Can you work these out from the model? Positions are in its coordinate system, mm. A direction names the side the tool comes from. Round coordinates to 2 decimals unless told otherwise and drop trailing zeros. Write each loop counter-clockwise with the first axis right and the second up, starting at its lowest first coordinate (ties: lowest second). Pieces come first, ordered by that corner, then holes. Notation, with made-up numbers: (48, 40) -> (83, 40) arc R19 cw to (83, 72) -> close; hole circle Ø7 at (33, -22.5). An arc over 180 degrees is marked (long way). Use CSV: the item, a comma, the result in double quotes.
Autodesk Inventor part; units mm, degrees
ref_plane "Work Plane1" through (64.0234, 0, 0) normal (0, 1, 0) x (-1, 0, 0)
ref_plane "YZ Plane" through (0, 0, 0) normal (1, 0, 0) x (0, 1, 0)
ref_plane "XZ Plane" through (0, 0, 0) normal (0, 1, 0) x (-1, 0, 0)
sketch "Sketch1" plane through (0, 0, 0) normal (0, 0, 1) x (1, 0, 0)
  line L0 (0, 0) -> (7, 0)
  line L1 (0, 0) -> (0, 22.5)
  line L2 (0, 22.5) -> (7, 22.5)
  line L3 (7, 22.5) -> (7, 0)
  line L4 (0, 27) -> (0, -4.5)
  line L5 (-1.4, 0) -> (8.4, 0)
  dimension "d1" = 45
  dimension "d2" = 7
revolve "Body" add sketch "Sketch1" angle 360 about axis through (0, 0, 0) along (1, 0, 0)
sketch "Sketch2" plane through (0, 0, 0) normal (-1, 0, 0) x (0, 0, 1)
  circle A0 centre (0, 0) radius 22.5
  point P0 (0, 0)
hole "Thread" at (0, 0, 0) direction (1, 0, 0) diameter 28.376 end through all
chamfer "Chamfer1" distance 3.5 angle 30 1 edges at (0, -22.5, 0) measured on face at (0, 19.4769, -2.3649)
sketch "Sketch3" plane through (7, 0, 0) normal (1, 0, 0) x (0, 0, -1)
  circle A0 centre (0, 0) radius 22.5
  line L0 (-2.5, 22.3607) -> (-2.5, 20.5)
  line L1 (-2.5, 20.5) -> (2.5, 20.5)
  line L2 (2.5, 20.5) -> (2.5, 22.3607)
  line L3 (0, -31.5) -> (0, 31.5)
  line L4 (-31.5, 0) -> (31.5, 0)
  dimension "d12" = 2.5
  dimension "d13" = 2.5
  dimension "d14" = 20.5
extrude "Groove1" cut sketch "Sketch3" against normal through all contours L2 L1 L3 A0 | L3 L1 L0 A0
pattern_circular "Grooves1" count 4 over 360 about axis through (-10, 0, 0) along (1, 0, 0) of "Groove1"
fillet "Fillet1" radius 0.7 4 edges at (7, 15.9099, 15.9099) (7, 15.9099, -15.9099) (7, -15.9099, -15.9099) (7, -15.9099, 15.9099)
chamfer "Chamfer2" distance 0.75 angle 45 1 edges at (7, 0, -14.188) measured on face at (7, 17.4258, 7.9613)
chamfer "Chamfer3" distance 0.75 angle 45 1 edges at (0, 0, -14.188) measured on face at (0, 17.1775, -2.0857)
ref_plane "Work Plane1" through (64.0234, 0, 0) normal (0, 1, 0) x (-1, 0, 0)
equation "\"d1\" = SD2"
equation "\"d2\" = KOH"
equation "\"d12\" = 0.5 * SNB"
equation "\"d13\" = 0.5 * SNB"
equation "\"d14\" = 0.5 * SD2 - SNT"
equation "\"d10\" = -0.5 * LADI + 0.5 * SD2"
equation "\"d11\" = FAWI2"
equation "\"d40\" = -0.5 * LADI + 0.5 * SD2"
equation "\"d18\" = RR"
equation "\"d19\" = 0.025 * NND"
equation "\"d41\" = 0.025 * NND"
equation "\"d21\" = 0.025 * NND"
equation "\"d42\" = 0.025 * NND"
equation "\"KOH\" = 7"
equation "\"SD2\" = 45"
equation "\"SNB\" = 5"
equation "\"SNT\" = 2"
equation "\"LADI\" = 38"
equation "\"RR\" = 0.1 * KOH"
equation "\"FAWI2\" = 30deg"
equation "\"GUL\" = 0.541266 * PTC"
equation "\"TOA\" = 30deg"
equation "\"PTC\" = 1.5"
equation "\"GAL\" = 0.541266 * PTC"
properties part number "ANSI/AFBMA Std 8.1 - KM 6" material "Steel, Mild"
Q1. If we mould it in two halves opening along Z, with no side actions, what happens to faces 1 (the face through (4, 2.5, 21)), 2 (the face through (4, -20.5, 0)), 3 (the face through (4.19, -15.76, 16.06))? For each: released by +Z, released by -Z, zero draft, split by the parting line, or undercut.
Resolved:
face 1,"zero draft"
face 2,"undercut"
face 3,"released by +Z"
Q2. Please list where these lines run through material, in increasing order: probe 1 along Z at (x, y) = (4.8, 0); probe 2 along Z at (x, y) = (2.5, 2).
Resolved:
probe 1,"z = -20.5 to -14.19, 14.19 to 20.5"
probe 2,"z = -20.5 to -14.05, 14.05 to 20.5"
Q3. On a 3-axis mill with a long thin cutter (end or side, diameter ignored), from which of +Z, -Z, +X, -X, +Y, -Y can I reach the whole of each face in a straight line? I mean faces 4 (the face through (4, -21, -2.5)), 5 (the face through (4, -2.5, 21)), 6 (the face through (4, 21, 2.5)). Say none if no direction works.
Resolved:
face 4,"+X, -X, -Y"
face 5,"+Z, +X, -X"
face 6,"+X, -X, +Y"
Q4. Will these pins go through, and if not, where does the flat tip stop? P1, Ø1, axis at x = 4, y = -7.5, coming from the +Z side; P2, Ø4, axis at x = 4, z = -12, coming from the -Y side; P3, Ø22.5, axis at y = 0, z = 0, coming from the +X side; P4, Ø1, axis at y = -13.5, z = -4, coming from the -X side.
Resolved:
P1,"stops at z = 21.38"
P2,"stops at y = -20.16"
P3,"passes through"
P4,"stops at x = 0.36"
Q5. Suppose I cut it at A-A (z = 0). Write out the boundary of the cut face in (x, y).
Resolved:
outline,"(0, -19) -> (0.87, -20.5) -> (7, -20.5) -> (7, -14.94) -> (6.25, -14.19) -> (0.75, -14.19) -> (0, -14.94) -> close; (0, 14.94) -> (0.75, 14.19) -> (6.25, 14.19) -> (7, 14.94) -> (7, 20.5) -> (0.87, 20.5) -> (0, 19) -> close"
